```python
from build123d import *

# Parameters (mm, degrees)
F0_W           = 400
F0_H           = 400
F1_DEPTH       = 40
F3_D           = 14
F3_CBORE_D     = 25.5
F3_CBORE_DEPTH = 20


with BuildPart() as f1:
    # F0 (on Front) → F1 (new body)
    with BuildSketch(Plane.XZ):
        with Locations((200, 200)):
            Rectangle(F0_W, F0_H)
    extrude(amount=F1_DEPTH)

    # F3 (through all)
    with Locations(Plane.XZ.offset(40)):
        with Locations((20, 380), (380, 380), (380, 20), (20, 20)):
            CounterBoreHole(F3_D / 2, F3_CBORE_D / 2, F3_CBORE_DEPTH)


solid = f1.part
```
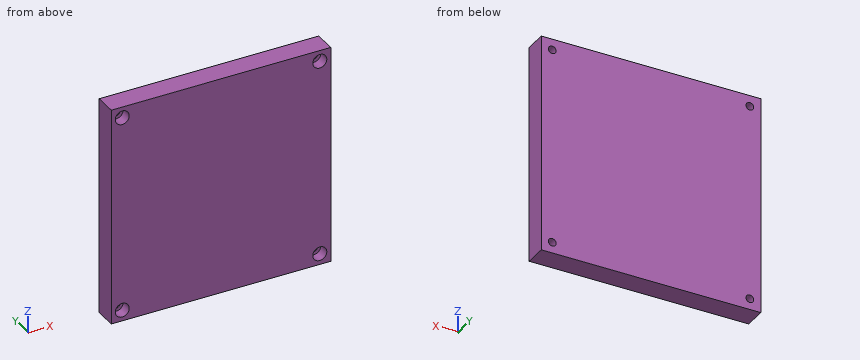
The listing builds one solid part. Answer for the finished solid, in the listing's coordinates (mm). Give positions to 0.01 mm unless a question says otherwise; leave off trailing zeros. Order: outer loops, then holes, each group sorted by start corner. A loop starts at its lowest first (then second) coordinate and runs counter-clockwise, first axis right, second up. Notation, with made-up numbers: (-13, 47) -> (14, 47) arc R17 ccw to (14, 72) -> close; hole circle Ø6 at (29.5, 86). An arc over 180 degrees is marked (long way). Write each question's results on one line, items separated by ' | '.
Q1. The part is cut by section B-B, the plane z = 20. Give the vertices of the cut face in (x, y).
Checked values:
outline: (0, -40) -> (7.25, -40) -> (7.25, -20) -> (13, -20) -> (13, 0) -> (0, 0) -> close; (27, -20) -> (32.75, -20) -> (32.75, -40) -> (367.25, -40) -> (367.25, -20) -> (373, -20) -> (373, 0) -> (27, 0) -> close; (387, -20) -> (392.75, -20) -> (392.75, -40) -> (400, -40) -> (400, 0) -> (387, 0) -> close
Q2. The part is cut by section A-A, the plane x = 20. Give the vertices of the cut face in (y, z), and give its area (3 significant figures).
Checked values:
outline: (-40, 0) -> (0, 0) -> (0, 13) -> (-20, 13) -> (-20, 7.25) -> (-40, 7.25) -> close; (-40, 32.75) -> (-20, 32.75) -> (-20, 27) -> (0, 27) -> (0, 373) -> (-20, 373) -> (-20, 367.25) -> (-40, 367.25) -> close; (-40, 392.75) -> (-20, 392.75) -> (-20, 387) -> (0, 387) -> (0, 400) -> (-40, 400) -> close | area: 14,400 mm^2
Q3. Straight lines are drawn through the part: probe 1 along Z at (x, y) = (20, -13.5); probe 2 along Z at (x, y) = (380, -27). For each, find the intervals that lie inside material, in ascending order. Write a range as from..to.
Checked values:
probe 1: z = 0..13, 27..373, 387..400 | probe 2: z = 0..7.25, 32.75..367.25, 392.75..400
Q4. Each of these flat-tipped pins is pushed along its axis until it touches: P1, Ø20.5, axis at x = 17, z = 378, coming from the -Y side; P2, Ø16, axis at x = 380, z = 380, coming from the -Y side. Where does it stop, or does it pass through?
Checked values:
P1: stops at y = -40 | P2: stops at y = -20
